from build123d import *

# Parameters (mm, degrees)
SKETCH1_W           = 140
SKETCH1_H           = 80
BOSS_EXTRUDE1_DEPTH = 2
SKETCH3_W           = 126
SKETCH3_H           = 66
SKETCH2_W           = 140
SKETCH2_H           = 80
CHAMFER2_SIZE       = 2
SKETCH4_W           = 8
SKETCH4_H           = 10
BOSS_EXTRUDE2_DEPTH = 7
SKETCH5_R           = 2.05
CUT_EXTRUDE1_DEPTH  = 133.9000001
SKETCH6_W           = 107.8
SKETCH6_H           = 64
CUT_EXTRUDE2_DEPTH  = 5


with BuildPart() as part:
    # Sketch1 → Boss-Extrude1 (new body)
    with BuildSketch(Plane(origin=(0, 0, 0), x_dir=(1, 0, 0), z_dir=(0, 1, 0))):
        Rectangle(SKETCH1_W, SKETCH1_H)
    extrude(amount=BOSS_EXTRUDE1_DEPTH)

    # Sketch3 → Loft1 section 0
    with BuildSketch(Plane(origin=(0, 7, 0), x_dir=(1, 0, 0), z_dir=(0, 1, 0))):
        Rectangle(SKETCH3_W, SKETCH3_H)
    # Sketch2 → Loft1 section 1
    with BuildSketch(Plane(origin=(0, 2, 0), x_dir=(1, 0, 0), z_dir=(0, 1, 0))):
        Rectangle(SKETCH2_W, SKETCH2_H)
    loft()

    # Chamfer2
    chamfer2_edges = [part.edges().sort_by_distance(p)[0] for p in [
        (70, 1, 40),
        (-70, 1, 40),
        (-70, 1, -40),
        (70, 1, -40),
    ]]
    chamfer(chamfer2_edges, length=CHAMFER2_SIZE)

    # Sketch4 → Boss-Extrude2 (add)
    with BuildSketch(Plane.XZ):
        with Locations((-58.9, 20)):
            Rectangle(SKETCH4_W, SKETCH4_H)
        with Locations((-58.9, -20)):
            Rectangle(SKETCH4_W, SKETCH4_H)
        with Locations((58.9, -20)):
            Rectangle(SKETCH4_W, SKETCH4_H)
        with Locations((58.9, 20)):
            Rectangle(SKETCH4_W, SKETCH4_H)
    extrude(amount=BOSS_EXTRUDE2_DEPTH)

    # Sketch5 → Cut-Extrude1 (cut, through all)
    with BuildSketch(Plane.ZY.offset(62.9)):
        with Locations((-20, -3.5)):
            Circle(SKETCH5_R)
        with Locations((20, -3.5)):
            Circle(SKETCH5_R)
    extrude(amount=-CUT_EXTRUDE1_DEPTH, mode=Mode.SUBTRACT)

    # Sketch6 → Cut-Extrude2 (cut)
    with BuildSketch(Plane.XZ):
        Rectangle(SKETCH6_W, SKETCH6_H)
    extrude(amount=-CUT_EXTRUDE2_DEPTH, mode=Mode.SUBTRACT)


solid = part.part
The model under review builds one solid part; all positions refer to its coordinate system, in mm. A direction names the side the tool comes from. Give positions to 0.01 mm unless a question says otherwise; leave off trailing zeros. Use one line per item in the form item = value. Start each with the question number.
Item 1: Insertion check: pin 1 Ø3.5 at (x, y) = (-57, -2.5) entering from -Z; pin 2 Ø5 at (x, y) = (-51, -3) entering from -Z; pin 3 Ø5 at (y, z) = (5, 21) entering from +X; pin 4 Ø3.5 at (y, z) = (-3.5, -19.5) entering from +X. Each pin has a flat end and moves straight along its axis. Give the tip position at first contact, or say it passes through.
Item 2: For faces 1 (the flat face through (-59, -3, -15)), 2 (the flat face through (54.9, -3.5, 17.7)), 3 (the flat face through (-1, 2, 32)), list the 3-axis set-ups (+Z, -Z, +X, -X, +Y, -Y) from which the entire face can be reached by the end or side of a thin tool; tool diameter is ignored.
Item 3: We need section A-A on y = -3.5. Give the number of separate pieces and of enclosed holes in the cut face, plus the area to 3 significant figures.
Item 4: The part is to be moulded in two halves that separate along Z. For faces 4 (the flat face through (59, -3, -25)), 5 (the flat face through (-1, 2, -32)), 6 (the flat face through (62.9, -3.5, -22.3)), say which applies: pulls with the +Z half, pulls with the -Z half, needs draft (parallel to the pull), parting line crosses it, or undercut.
Item 5: To check wall thickness, follow line 1 along Y through (x, z) = (-58, -20); line 2 along Z through (x, y) = (-36.5, 0.75); line 3 along X through (y, z) = (2, 0). State the ranges of each line that lie inside material, in increasing order. Write a range as from..to.
Completed:
q1.pin_1 = -25
q1.pin_2 = through
q1.pin_3 = 69.3
q1.pin_4 = 62.9
q2.face_1 = +X, -X, -Y
q2.face_2 = +Z, -Z, -Y
q2.face_3 = -Y
q3.separate_pieces = 8
q3.enclosed_holes = 0
q3.area = 189 mm²
q4.face_4 = pulls with the -Z half
q4.face_5 = undercut
q4.face_6 = needs draft
q5.line_1 = -7..-5.55, -1.45..7
q5.line_2 = -40..-32, 32..40
q5.line_3 = -70..-53.9, 53.9..70
